Study the drawing (mm; zero at the part's minimum x, y, z) and answer. A direction names the side the tool comes from. Round coordinates to 2 decimals unless told otherwise and drop trailing zeros. Loops run counter-clockwise (first coordinate to the right, second up) from the corner with the lowest first, then second, coordinate; pieces in that order, holes last. Notation, with made-up numbers: M 80,33 L 104,33 A12 cw 104,47 Z; hole C -31.75,18 d4. An arc over 180 degrees is marked long. Write each question's results on one line, items separated by ' | '.
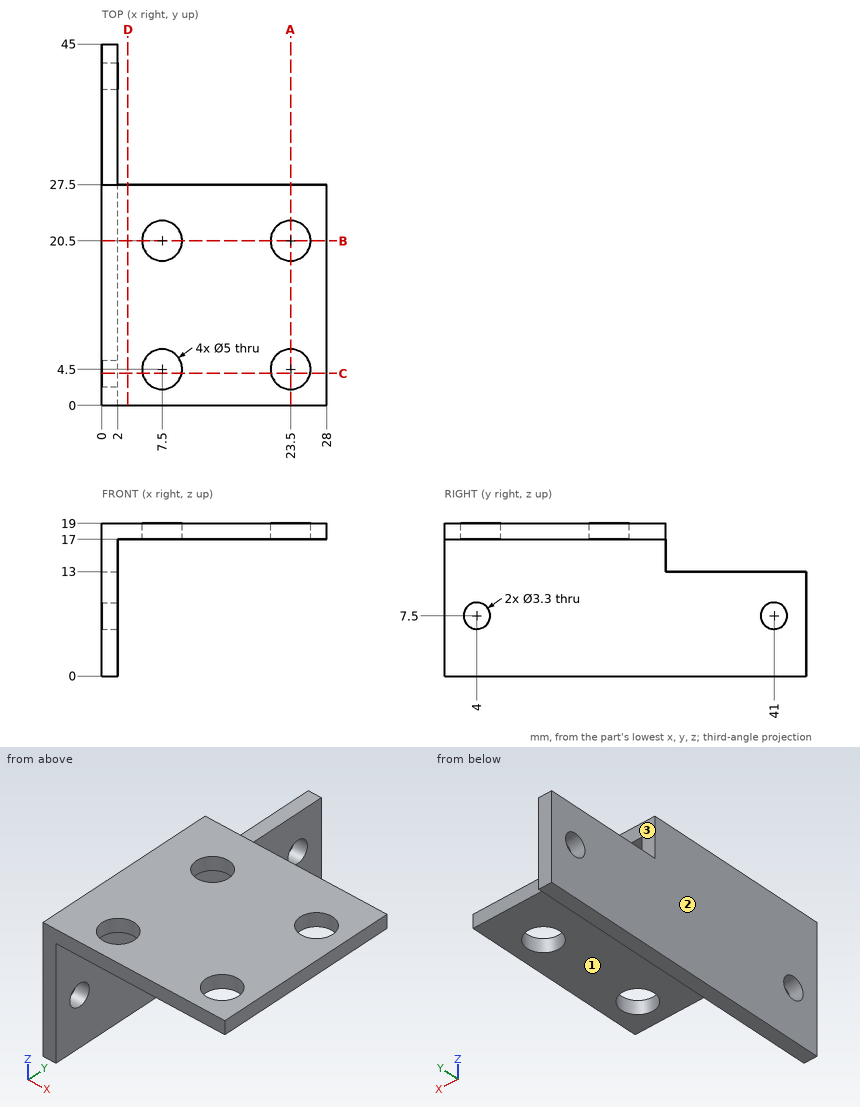
Item 1: Straight lines are drawn through the part: line 1 (X direction, y = 20.5, z = 18.6); line 2 (Y direction, x = 7.5, z = 18.2); line 3 (X direction, y = 6.5, z = 17.25). For each, find the intervals that lie inside material, in ascending order.
Outcome:
line 1: x = 0 to 5, 10 to 21, 26 to 28 | line 2: y = 0 to 2, 7 to 18, 23 to 27.5 | line 3: x = 0 to 6, 9 to 22, 25 to 28
Item 2: Flat-ended cylindrical pins translate along their axes: pin 1 (2 mm diameter, centred on x = 10, y = 26.5, fed in from -Z); pin 2 (6 mm diameter, centred on x = 6.5, y = 31.5, fed in from +Z); pin 3 (5.5 mm diameter, centred on y = 41, z = 7.5, fed in from +X); pin 4 (6.5 mm diameter, centred on x = 19.5, z = 15.5, fed in from +Y). Find the tip coordinate at first contact, or state that the pin passes through.
Outcome:
pin 1: stops at z = 17 | pin 2: passes through | pin 3: stops at x = 2 | pin 4: stops at y = 27.5
Item 3: The part is cut by section C-C (y = 4). Determine the outline of the cut face in (x, z).
Outcome:
outline: M 0,0 L 2,0 L 2,5.85 L 0,5.85 Z; M 0,9.15 L 2,9.15 L 2,17 L 5.05,17 L 5.05,19 L 0,19 Z; M 9.95,17 L 21.05,17 L 21.05,19 L 9.95,19 Z; M 25.95,17 L 28,17 L 28,19 L 25.95,19 Z
Item 4: For the marked faces 1, 2 and 3, determine the directions among +Z, -Z, +X, -X, +Y, -Y from which every point of the face is accessible in a straight line to the end or side of a thin tool.
Outcome:
face 1: -Z, +X, +Y, -Y | face 2: +Z, -Z, -X, +Y, -Y | face 3: +Z, +X, -X, +Y
Item 5: The part is cut by section D-D (x = 3.25). Determine the outline of the cut face in (y, z), plus the area to 3 significant figures.
Outcome:
outline: M 0,17 L 27.5,17 L 27.5,19 L 0,19 Z | area: 55.0 mm2
Item 6: The part is cut by section A-A (x = 23.5). Determine the outline of the cut face in (y, z), plus the area to 3 significant figures.
Outcome:
outline: M 0,17 L 2,17 L 2,19 L 0,19 Z; M 7,17 L 18,17 L 18,19 L 7,19 Z; M 23,17 L 27.5,17 L 27.5,19 L 23,19 Z | area: 35.0 mm2
Item 7: The part is cut by section B-B (y = 20.5). Determine the outline of the cut face in (x, z).
Outcome:
outline: M 0,0 L 2,0 L 2,17 L 5,17 L 5,19 L 0,19 Z; M 10,17 L 21,17 L 21,19 L 10,19 Z; M 26,17 L 28,17 L 28,19 L 26,19 Z
